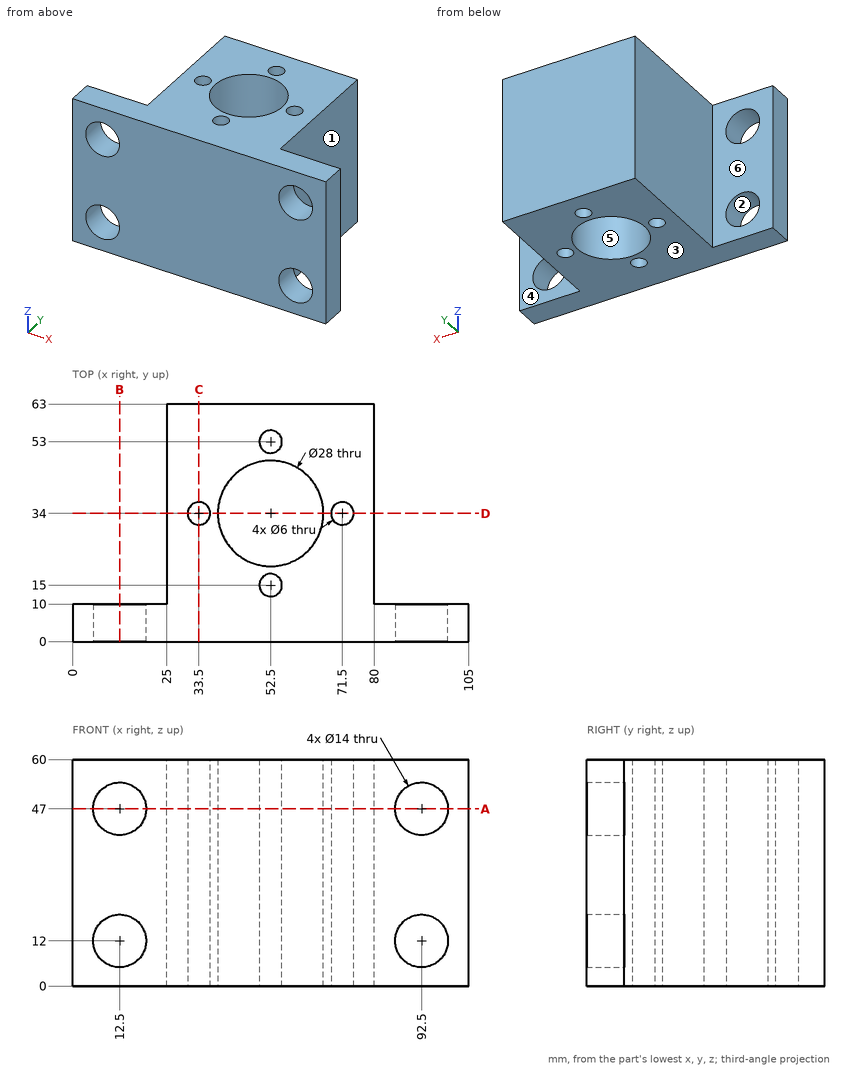
Geometry: see drawing. Coordinates: mm, zero at the bounding-box minimum. A direction names the side the tool comes from. Give positions to 0.01 mm unless a question says otherwise; leave off trailing zeros. Loops run counter-clockwise (first coordinate to the right, second up) from the corner with the lowest first, then second, coordinate; pieces in that order, holes last. Notation, with made-up numbers: (73, 26) - (120, 26) arc R26 cw to (120, 46) - close; hole circle Ø1 at (65, 70). An arc over 180 degrees is marked (long way). Use CSV: the item, a comma, the result in double quotes. Start each with the question number.
1. Section B-B (x = 12.5). Output: boundary loops of the cut face in (y, z).
2. Ray query, L1, parallel to Z at x = 12, y = 3; L2, parallel to Y at x = 52.5, z = 14.5; L3, parallel to X at y = 31.5, z = 27. Return the intervals inside material, ascending.
3. Reachability of the marked faces 4, 5 and 6 from +Z, -Z, +X, -X, +Y, -Y: full face, straight path, thin tool, end or side. Return the list, or none.
4. Section A-A (z = 47). Output: boundary loops of the cut face in (x, y).
5. Section D-D (y = 34). Output: boundary loops of the cut face in (x, z).
6. Draft query along Z for the marked faces 1, 2 and 3. Return one class per face: +Z half, -Z half, draft (parallel to the pull), parting line (faces both ways), or undercut.
7. Section C-C (x = 33.5). Output: boundary loops of the cut face in (y, z).
8. Pin query (flat end, axial travel): pin 1 (10 mm diameter, centred on y = 18, z = 23.5, fed in from +X); pin 2 (22.5 mm diameter, centred on x = 12.5, z = 12, fed in from +Y); pin 3 (11 mm diameter, centred on x = 12.5, z = 47, fed in from +Y); pin 4 (10 mm diameter, centred on y = 26, z = 36, fed in from -X). Return the tip coordinate at first contact, or that it passes through.
Response:
1,outline,"(0, 0) - (10, 0) - (10, 5) - (0, 5) - close; (0, 19) - (10, 19) - (10, 40) - (0, 40) - close; (0, 54) - (10, 54) - (10, 60) - (0, 60) - close"
2,L1,"0 to 5.02, 18.98 to 40.02, 53.98 to 60"
2,L2,"0 to 12, 18 to 20, 48 to 50, 56 to 63"
2,L3,"25 to 31.84, 35.16 to 38.73, 66.27 to 69.84, 73.16 to 80"
3,face 4,"+Z, -Z, +X, +Y"
3,face 5,"+Z, -Z"
3,face 6,"+Z, -Z, -X, +Y"
4,outline,"(0, 0) - (5.5, 0) - (5.5, 10) - (0, 10) - close; (19.5, 0) - (85.5, 0) - (85.5, 10) - (80, 10) - (80, 63) - (25, 63) - (25, 10) - (19.5, 10) - close; (99.5, 0) - (105, 0) - (105, 10) - (99.5, 10) - close; hole circle Ø6 at (33.5, 34); hole circle Ø28 at (52.5, 34); hole circle Ø6 at (52.5, 15); hole circle Ø6 at (52.5, 53); hole circle Ø6 at (71.5, 34)"
5,outline,"(25, 0) - (30.5, 0) - (30.5, 60) - (25, 60) - close; (36.5, 0) - (38.5, 0) - (38.5, 60) - (36.5, 60) - close; (66.5, 0) - (68.5, 0) - (68.5, 60) - (66.5, 60) - close; (74.5, 0) - (80, 0) - (80, 60) - (74.5, 60) - close"
6,face 1,"draft"
6,face 2,"undercut"
6,face 3,"-Z half"
7,outline,"(0, 0) - (31, 0) - (31, 60) - (0, 60) - close; (37, 0) - (63, 0) - (63, 60) - (37, 60) - close"
8,pin 1,"x = 80"
8,pin 2,"y = 10"
8,pin 3,"through"
8,pin 4,"x = 25"
